The listing builds one solid part. Answer for the finished solid, in the listing's coordinates (mm). A direction names the side the tool comes from. Round coordinates to 2 decimals unless told otherwise and drop trailing zeros. Write each loop counter-clockwise with the first axis right and the second up, starting at its lowest first coordinate (ties: lowest second). Pieces come first, ordered by that corner, then holes. Notation, with made-up numbers: (-1, 84.25) - (5, 84.25) arc R16 ccw to (5, 99.25) - close; hole circle Ø3 at (50.25, -34). An arc over 180 degrees is marked (long way). Answer in a Markdown table with one row per item.
from build123d import *

# Parameters (mm, degrees)
F1_DEPTH      = 2700
F3_DEPTH      = 159
F5_W          = 67
F5_H          = 56.321
F6_DEPTH      = 25
F8_DEPTH      = 192.001
F8_DEPTH_BACK = 39.001


with BuildPart() as f1:
    # F0 (on Top) → F1 (new body)
    with BuildSketch(Plane.XY):
        with BuildLine():
            Line((-44.5896353125, 6), (-44.5896353125, 0))
            Line((-44.5896353125, 0), (22.4103646875, 0))
            ThreePointArc((22.4103646875, 0), (28.067218937, -2.3431457505), (30.4103646875, -8))
            Line((30.4103646875, -8), (30.4103646875, -31))
            ThreePointArc((30.4103646875, -31), (32.753510438, -36.6568542495), (38.4103646875, -39))
            Line((38.4103646875, -39), (193.4103646875, -39))
            ThreePointArc((193.4103646875, -39), (199.067218937, -36.6568542495), (201.4103646875, -31))
            Line((201.4103646875, -31), (201.4103646875, 109))
            ThreePointArc((201.4103646875, 109), (199.067218937, 114.6568542495), (193.4103646875, 117))
            Line((193.4103646875, 117), (159.4103646875, 117))
            ThreePointArc((159.4103646875, 117), (153.753510438, 119.3431457505), (151.4103646875, 125))
            Line((151.4103646875, 125), (151.4103646875, 192))
            Line((151.4103646875, 192), (145.4103646875, 192))
            Line((145.4103646875, 192), (145.4103646875, 119))
            ThreePointArc((145.4103646875, 119), (147.753510438, 113.3431457505), (153.4103646875, 111))
            Line((153.4103646875, 111), (187.4103646875, 111))
            ThreePointArc((187.4103646875, 111), (193.067218937, 108.6568542495), (195.4103646875, 103))
            Line((195.4103646875, 103), (195.4103646875, -25))
            ThreePointArc((195.4103646875, -25), (193.067218937, -30.6568542495), (187.4103646875, -33))
            Line((187.4103646875, -33), (44.4103646875, -33))
            ThreePointArc((44.4103646875, -33), (38.753510438, -30.6568542495), (36.4103646875, -25))
            Line((36.4103646875, -25), (36.4103646875, -2))
            ThreePointArc((36.4103646875, -2), (34.067218937, 3.6568542495), (28.4103646875, 6))
            Line((28.4103646875, 6), (-44.5896353125, 6))
        make_face()
    extrude(amount=F1_DEPTH)

    # F2 (on face) → F3 (cut)
    with BuildSketch(Plane.XZ.offset(39)):
        Polygon((201.4103646875, 0), (201.4103646875, 20), (193.4103646875, 20), (26.4103646875, 20), (26.4103646875, 0), (38.4103646875, 0), (193.4103646875, 0), align=None)
        Polygon((193.4103646875, 2700), (38.4103646875, 2700), (26.4103646875, 2700), (26.4103646875, 2680), (193.4103646875, 2680), (201.4103646875, 2680), (201.4103646875, 2700), align=None)
    extrude(amount=-F3_DEPTH, mode=Mode.SUBTRACT)

    # F5 (on face) → F6 (cut)
    with BuildSketch(Plane(origin=(145.4103646875, 0, 0), x_dir=(0, -1, 0), z_dir=(-1, 0, 0))):
        with Locations((-158.5, 28.1605)):
            Rectangle(F5_W, F5_H)
    extrude(amount=-F6_DEPTH, mode=Mode.SUBTRACT)

    # F7 (on Front) → F8 (cut, two sides)
    with BuildSketch(Plane.XZ) as f8_sk:
        Polygon((-44.5896353125, 62), (-44.5896353125, 0), (22.4103646875, 0), (26.4103646875, 0), (26.4103646875, 20), (26.4103646875, 62), align=None)
    extrude(amount=-F8_DEPTH, mode=Mode.SUBTRACT)
    extrude(f8_sk.sketch, amount=F8_DEPTH_BACK, mode=Mode.SUBTRACT)


solid = f1.part
(1) Section B-B (x = -12.5) is taken. Give the vertices of the cut face in (y, z).
Checked values:
| item | result |
|---|---|
| outline | (0, 62) - (6, 62) - (6, 2700) - (0, 2700) - close |
(2) For a pull along Y with two mould halves and no side action, classify faces 1 (the flat face through (146, -36, 2680)), 2 (the flat face through (117, -33, 1331)), 3 (the flat face through (-12, 0, 1363)) as pulls with the +Y half, pulls with the -Y half, needs draft (parallel to the pull), parting line crosses it, or undercut.
Checked values:
| item | result |
|---|---|
| face 1 | needs draft |
| face 2 | undercut |
| face 3 | pulls with the -Y half |
(3) Section A-A (z = 225) is taken. Give the vertices of the cut face in (x, y).
Checked values:
| item | result |
|---|---|
| outline | (-44.59, 0) - (22.41, 0) arc R8 cw to (30.41, -8) - (30.41, -31) arc R8 ccw to (38.41, -39) - (193.41, -39) arc R8 ccw to (201.41, -31) - (201.41, 109) arc R8 ccw to (193.41, 117) - (159.41, 117) arc R8 cw to (151.41, 125) - (151.41, 192) - (145.41, 192) - (145.41, 119) arc R8 ccw to (153.41, 111) - (187.41, 111) arc R8 cw to (195.41, 103) - (195.41, -25) arc R8 cw to (187.41, -33) - (44.41, -33) arc R8 cw to (36.41, -25) - (36.41, -2) arc R8 ccw to (28.41, 6) - (-44.59, 6) - close |
(4) Flat-ended cylindrical pins translate along their axes: pin 1 (5 mm diameter, centred on y = 37, z = 406, fed in from -X); pin 2 (11.5 mm diameter, centred on y = -14.5, z = 769, fed in from -X); pin 3 (8 mm diameter, centred on y = 4, z = 2686, fed in from +X); pin 4 (3 mm diameter, centred on x = 151.5, y = 136, fed in from +Z). Find the tip coordinate at first contact, or state that the pin passes through.
Checked values:
| item | result |
|---|---|
| pin 1 | stops at x = 195.41 |
| pin 2 | stops at x = 30.41 |
| pin 3 | stops at x = 26.41 |
| pin 4 | stops at z = 2700 |
(5) Find the intervals of material crossed by line 1 (Y direction, x = 157, z = 592); line 2 (X direction, y = -6.5, z = 1273); line 3 (Y direction, x = 151, z = 562), in increasing order.
Checked values:
| item | result |
|---|---|
| line 1 | y = -39 to -33, 111 to 117.37 |
| line 2 | x = 30.27 to 36.41, 195.41 to 201.41 |
| line 3 | y = -39 to -33, 111.37 to 192 |
(6) For faces 4 (the flat face through (145.41, 156, 1331)), 5 (the flat face through (151.41, 158, 1360)), 6 (the flat face through (195.41, 40, 1331)), determine the directions among +Z, -Z, +X, -X, +Y, -Y from which every point of the face is accessible in a straight line to the end or side of a thin tool.
Checked values:
| item | result |
|---|---|
| face 4 | +Z, -Z, -X, +Y |
| face 5 | +Z, -Z, +X, +Y |
| face 6 | +Z, -Z |
